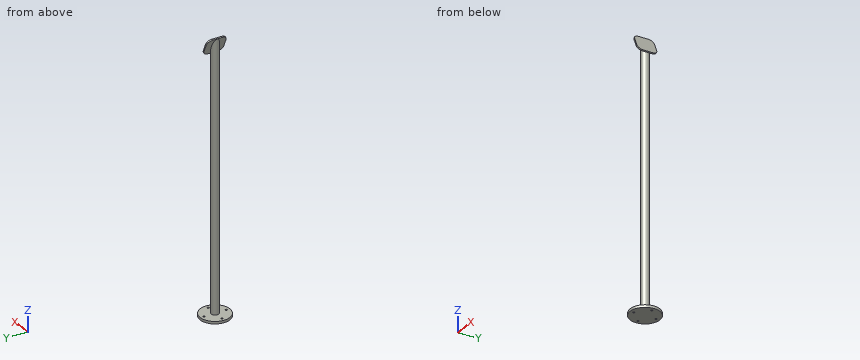
from build123d import *

# Parameters (mm, degrees)
SKETCH1_R           = 60
SKETCH1_R_2         = 4
BOSS_EXTRUDE1_DEPTH = 10
SKETCH2_R           = 15
BOSS_EXTRUDE2_DEPTH = 1080
CUT_EXTRUDE1_REACH  = 1017.827
SKETCH4_W           = 30
SKETCH4_H           = 150
BOSS_EXTRUDE3_DEPTH = 5


with BuildPart() as part:
    # Sketch1 → Boss-Extrude1 (new body)
    with BuildSketch(Plane.XY):
        Circle(SKETCH1_R)
        with Locations((0, 45)):
            Circle(SKETCH1_R_2, mode=Mode.SUBTRACT)
        with Locations((45, 0)):
            Circle(SKETCH1_R_2, mode=Mode.SUBTRACT)
        with Locations((0, -45)):
            Circle(SKETCH1_R_2, mode=Mode.SUBTRACT)
        with Locations((-45, 0)):
            Circle(SKETCH1_R_2, mode=Mode.SUBTRACT)
    extrude(amount=BOSS_EXTRUDE1_DEPTH)

    # Sketch2 → Boss-Extrude2 (add)
    with BuildSketch(Plane.XY.offset(10)):
        Circle(SKETCH2_R)
    extrude(amount=BOSS_EXTRUDE2_DEPTH)

    # Sketch4 → Cut-Extrude1 (cut, up to next)
    with BuildSketch(Plane(origin=(405.173314427, 0, 188.935419397), x_dir=(0, -1, 0), z_dir=(0.906307787036651, 0, 0.4226182617406972)), mode=Mode.PRIVATE) as cut_extrude1_sk1:
        with Locations((0, -987.87548787)):
            Rectangle(SKETCH4_W, SKETCH4_H)
    cut_extrude1_tool1 = extrude(cut_extrude1_sk1.sketch, amount=CUT_EXTRUDE1_REACH, mode=Mode.PRIVATE) & part.part
    add(cut_extrude1_tool1.solids().sort_by_distance((-12.320907, 0, 1084.254667))[0], mode=Mode.SUBTRACT)

    # Sketch5 → Boss-Extrude3 (add)
    with BuildSketch(Plane(origin=(405.173314427, 0, 188.935419397), x_dir=(0.42261826174069705, 0, -0.906307787036651), z_dir=(0.906307787036651, 0, 0.42261826174069705))):
        with BuildLine():
            Line((-941.221738049, -40), (-976.221738049, -40))
            ThreePointArc((-976.221738049, -40), (-990.363873672, -34.142135624), (-996.221738049, -20))
            Line((-996.221738049, -20), (-996.221738049, 20))
            ThreePointArc((-996.221738049, 20), (-990.363873672, 34.142135624), (-976.221738049, 40))
            Line((-976.221738049, 40), (-941.221738049, 40))
            ThreePointArc((-941.221738049, 40), (-927.079602425, 34.142135624), (-921.221738049, 20))
            Line((-921.221738049, 20), (-921.221738049, -20))
            ThreePointArc((-921.221738049, -20), (-927.079602425, -34.142135624), (-941.221738049, -40))
        make_face()
    extrude(amount=BOSS_EXTRUDE3_DEPTH)


solid = part.part
Can you work these out from the model? Positions are in its coordinate system, mm. Round coordinates to 2 decimals unless told otherwise and drop trailing zeros. Order: outer loops, then holes, each group sorted by start corner. A loop starts at its lowest first (then second) coordinate and runs counter-clockwise, first axis right, second up. Notation, with made-up numbers: (28.5, 11.5) - (43.5, 11.5) arc R16 cw to (43.5, 20.5) - close; hole circle Ø3 at (12.5, -38.5). An arc over 180 degrees is marked (long way). Answer in a Markdown table with one row per item.
(1) Suppose I cut it at B-B, the plane z = 605.5. Please give me the cut outline in (x, y), plus the area to 3 significant figures.
From the geometry:
| item | result |
|---|---|
| outline | circle Ø30 at (0, 0) |
| area | 707 mm2 |
(2) For P1, Ø8, axis at x = 41, y = 31, coming from the +Z side; P2, Ø6.5, axis at x = -45, y = 0, coming from the -Z side; P3, Ø6, axis at y = -15, z = 952.5, coming from the -X side; P4, Ø15.5, axis at x = 4, z = 1058.5, coming from the +Y side, each with a flat end and sliding along its axis, tell me the tip position at first contact or that it passes through.
From the geometry:
| item | result |
|---|---|
| P1 | stops at z = 10 |
| P2 | passes through |
| P3 | stops at x = -9 |
| P4 | stops at y = 40 |
(3) Please list where these lines run through material, in increasing order: L1, parallel to Y at x = 0, z = 7; L2, parallel to X at y = -1, z = 878.5; L3, parallel to Z at x = -16, y = -39. Write a range as from..to.
From the geometry:
| item | result |
|---|---|
| L1 | y = -60..-49, -41..41, 49..60 |
| L2 | x = -14.97..14.97 |
| L3 | z = 0..10 |
(4) Suppose I cut it at A-A, the plane y = 30. Please give me the cut outline in (x, z), plus the area to 3 significant figures.
From the geometry:
| item | result |
|---|---|
| outline | (-51.96, 0) - (51.96, 0) - (51.96, 10) - (-51.96, 10) - close; (-14.72, 1089.39) - (14.72, 1026.27) - (19.25, 1028.39) - (-10.18, 1091.5) - close |
| area | 1,390 mm2 |
